Geometry check sheet. Reference: drawing and pictorial views, mm from the part's lowest x, y, z. A direction names the side the tool comes from. Give positions to 0.01 mm unless a question says otherwise; leave off trailing zeros. Loops run counter-clockwise (first coordinate to the right, second up) from the corner with the lowest first, then second, coordinate; pieces in that order, holes last. Notation, with made-up numbers: M 77.25,31 L 111.25,31 A19 ccw 111.25,59 Z; hole C 50,67.25 d5. An arc over 180 degrees is marked long. Use CSV: the item, a comma, the result in double quotes.
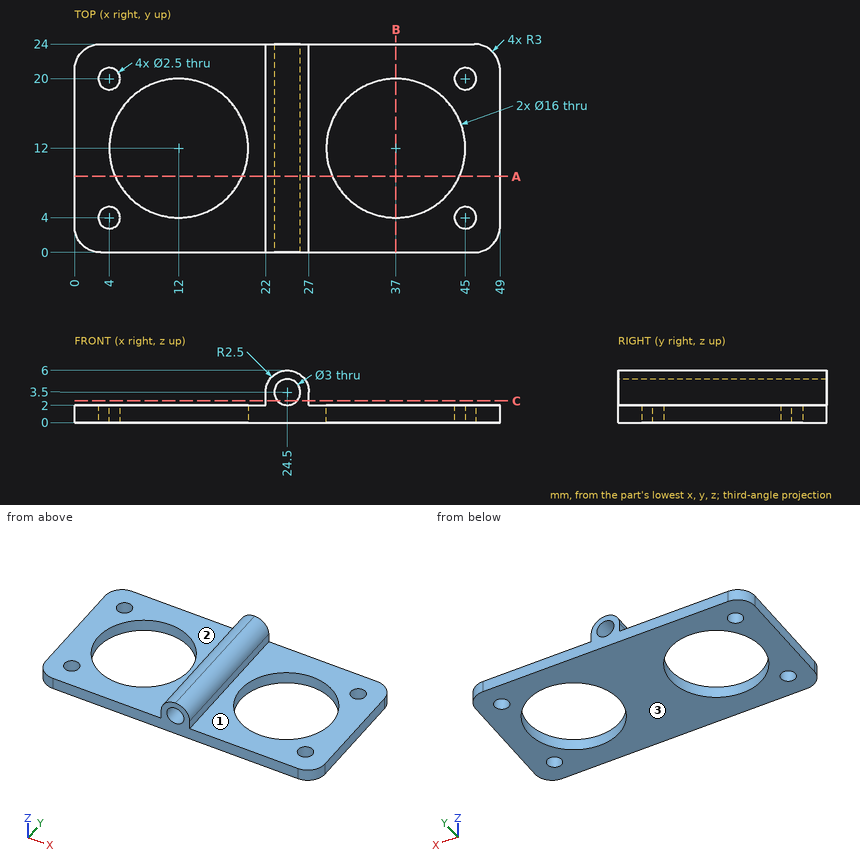
(1) Section check C-C on z = 2.5. Record the cut outline in (x, y), plus the area to 3 significant figures.
Calculated:
outline,"M 22,0 L 23.38,0 L 23.38,24 L 22,24 Z; M 25.62,0 L 27,0 L 27,24 L 25.62,24 Z"
area,"66.3 mm²"
(2) Section check B-B on x = 37. Record the cut outline in (y, z).
Calculated:
outline,"M 0,0 L 4,0 L 4,2 L 0,2 Z; M 20,0 L 24,0 L 24,2 L 20,2 Z"
(3) Scan lines: L1, parallel to X at y = 3.5, z = 1.75; L2, parallel to X at y = 10, z = 1.8; L3, parallel to Y at x = 12, z = 1.5. Record each from-to range of solid material in increasing order. Write a range as from..to.
Calculated:
L1,"x = 0..2.85, 5.15..43.85, 46.15..49"
L2,"x = 0..4.25, 19.75..29.25, 44.75..49"
L3,"y = 0..4, 20..24"
(4) Tool access check on the marked faces 1, 2 and 3. Record the directions out of +Z, -Z, +X, -X, +Y, -Y that give a thin tool (end or side, any length) a straight path to the whole face; none if there is none.
Calculated:
face 1,"+Z, +X, +Y, -Y"
face 2,"+Z, -X, +Y, -Y"
face 3,"-Z, +X, -X, +Y, -Y"
(5) Depth check by flat-ended pin: pin 1 Ø3 at (x, y) = (45, 4) entering from -Z; pin 2 Ø0.8 at (y, z) = (8.5, 2.5) entering from -X; pin 3 Ø3 at (x, y) = (4, 4) entering from +Z; pin 4 Ø0.5 at (y, z) = (6.5, 2.5) entering from +X. Enter the tip coordinate at first touch or a pass-through.
Calculated:
pin 1,"stops at z = 0"
pin 2,"stops at x = 22"
pin 3,"stops at z = 2"
pin 4,"stops at x = 27"
(6) Section check A-A on y = 8.75. Count the separate pieces of the cut face and the enclosed holes in it, plus the area to 3 significant figures.
Calculated:
separate pieces,"3"
enclosed holes,"1"
area,"49.8 mm²"
